Geometry: see drawing. Coordinates: mm, zero at the bounding-box minimum. Round coordinates to 2 decimals unless told otherwise and drop trailing zeros. Order: outer loops, then holes, each group sorted by start corner. A loop starts at its lowest first (then second) coordinate and runs counter-clockwise, first axis right, second up. Notation, with made-up numbers: M -35.75,79.5 L 8.25,79.5 A17 ccw 8.25,109.5 Z; hole C 76.5,23.25 d10. An arc over 180 degrees is marked long. Answer in a Markdown table with one row per item. Add a question column.
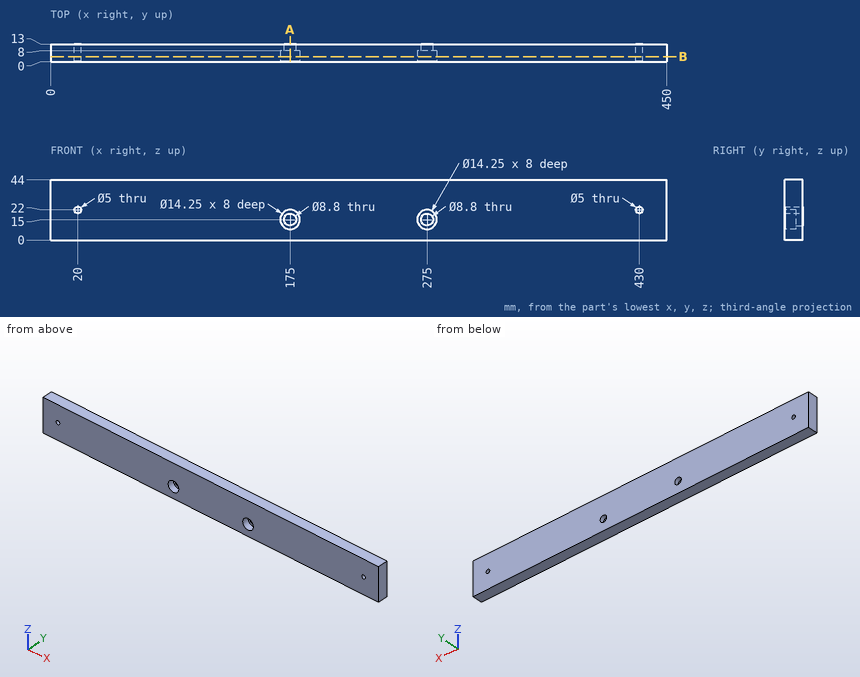
(1) Cut plane A-A (x = 175). Return loops of the section in (y, z) (3 decimals).
(2) Pin query (flat end, axial travel): pin 1 (16.5 mm diameter, centred on x = 275, z = 15, fed in from +Y); pin 2 (3 mm diameter, centred on x = 20, z = 22, fed in from +Y); pin 3 (11.5 mm diameter, centred on x = 275, z = 15.5, fed in from -Y). Return the tip coordinate at first contact, or that it passes through.
(3) Line query: line 1 (X direction, y = 10, z = 15.5); line 2 (Z direction, x = 275, y = 11.15); line 3 (X direction, y = 6.75, z = 23). Output: solid intervals per line, ascending. Write a range as from..to.
(4) Cut plane B-B (y = 3.75). Return loops of the section in (x, z) (3 decimals).
Answer list:
| question | item | result |
|---|---|---|
| 1 | outline | M 0,0 L 13,0 L 13,10.6 L 8,10.6 L 8,7.875 L 0,7.875 Z; M 0,22.125 L 8,22.125 L 8,19.4 L 13,19.4 L 13,44 L 0,44 Z |
| 2 | pin 1 | y = 13 |
| 2 | pin 2 | through |
| 2 | pin 3 | y = 8 |
| 3 | line 1 | 0..170.63, 179.37..270.63, 279.37..450 |
| 3 | line 2 | 0..10.6, 19.4..44 |
| 3 | line 3 | 0..17.71, 22.29..427.71, 432.29..450 |
| 4 | outline | M 0,0 L 450,0 L 450,44 L 0,44 Z; hole C 20,22 d5; hole C 175,15 d14.25; hole C 275,15 d14.25; hole C 430,22 d5 |
